The listing builds one solid part. Answer for the finished solid, in the listing's coordinates (mm). A direction names the side the tool comes from. Give positions to 0.01 mm unless a question says otherwise; leave off trailing zeros. Order: outer loops, then holes, each group sorted by start corner. A loop starts at its lowest first (then second) coordinate and runs counter-clockwise, first axis right, second up. Notation, with made-up numbers: (29.25, -29) - (73.25, -29) arc R20 cw to (73.25, -19) - close; hole circle Ø4 at (30, 65). An arc over 180 degrees is marked (long way). Use CSV: the item, a comma, the result in double quotes.
```python
from build123d import *

# Parameters (mm, degrees)
SKETCH1_W               = 140
SKETCH1_H               = 60
BOSS_EXTRUDE1_DEPTH     = 5
SKETCH2_W               = 140
SKETCH2_H               = 5
BOSS_EXTRUDE3_DEPTH     = 50
SKETCH4_R               = 7
CUT_EXTRUDE1_DEPTH      = 108.354552768
SKETCH5_W               = 50
SKETCH5_H               = 50
SKETCH5_W_2             = 40
SKETCH5_H_2             = 40
BOSS_EXTRUDE4_DEPTH     = 1015
CUT_EXTRUDE3_DEPTH      = 2088.648198332
CUT_EXTRUDE3_DEPTH_BACK = 2088.648198332


with BuildPart() as part:
    # Sketch1 → Boss-Extrude1 (new body)
    with BuildSketch(Plane(origin=(0, 0, 0), x_dir=(1, 0, 0), z_dir=(0, 1, 0))):
        with Locations((0, 15)):
            Rectangle(SKETCH1_W, SKETCH1_H)
    extrude(amount=-BOSS_EXTRUDE1_DEPTH)

    # Sketch2 → Boss-Extrude3 (add)
    with BuildSketch(Plane.XZ.offset(5)):
        with Locations((0, 12.5)):
            Rectangle(SKETCH2_W, SKETCH2_H)
        with Locations((0, -42.5)):
            Rectangle(SKETCH2_W, SKETCH2_H)
    extrude(amount=BOSS_EXTRUDE3_DEPTH)

    # Sketch4 → Cut-Extrude1 (cut, through all)
    with BuildSketch(Plane.XY.offset(15)):
        with Locations((-45, -27.5)):
            Circle(SKETCH4_R)
        with Locations((45, -27.5)):
            Circle(SKETCH4_R)
    extrude(amount=-CUT_EXTRUDE1_DEPTH, mode=Mode.SUBTRACT)

    # Sketch5 → Boss-Extrude4 (add)
    with BuildSketch(Plane(origin=(0, 0, 0), x_dir=(1, 0, 0), z_dir=(0, 1, 0))):
        with Locations((0, 15)):
            Rectangle(SKETCH5_W, SKETCH5_H)
        with Locations((0, 15)):
            Rectangle(SKETCH5_W_2, SKETCH5_H_2, mode=Mode.SUBTRACT)
    extrude(amount=BOSS_EXTRUDE4_DEPTH)

    # Mirror1: part across plane


with BuildPart() as part_1:
    add(part.part)
    add(part.part.mirror(Plane.ZX.offset(1015)))

    # Sketch8 → Cut-Extrude3 (cut, two sides: drawn at the far end of the back side and taken through both)
    with BuildSketch(Plane.ZY.offset(25).offset(-CUT_EXTRUDE3_DEPTH_BACK)):
        with BuildLine():
            Line((-32.587539874, 2030), (-32.587539874, 1955.085156016))
            ThreePointArc((-32.587539874, 1955.085156016), (-16.293769937, 1938.791386079), (0, 1955.085156016))
            Line((0, 1955.085156016), (0, 2030))
            Line((0, 2030), (-32.587539874, 2030))
        make_face()
    extrude(amount=CUT_EXTRUDE3_DEPTH + CUT_EXTRUDE3_DEPTH_BACK, mode=Mode.SUBTRACT)


solid = part_1.part
```
Item 1: The part is cut by section B-B (z = -17). Give the vertices of the cut face in (x, y), and give its area (3 significant figures).
Taken from the geometry:
outline,"(-70, -5) - (70, -5) - (70, 0) - (25, 0) - (25, 1938.81) - (20, 1938.81) - (20, 0) - (-20, 0) - (-20, 1938.81) - (-25, 1938.81) - (-25, 0) - (-70, 0) - close; (-70, 2030) - (70, 2030) - (70, 2035) - (-70, 2035) - close"
area,"20,800 mm^2"
Item 2: Find the intervals of material crossed by line 1 along Y through (x, z) = (-45, 12.45); line 2 along Z through (x, y) = (-8.5, 1957); line 3 along X through (y, z) = (736, -33), in increasing order.
Taken from the geometry:
line 1,"-55 to -34.5, -20.5 to 0, 2030 to 2050.5, 2064.5 to 2085"
line 2,"-40 to -35, 5 to 10"
line 3,"-25 to -20, 20 to 25"
Item 3: Each of these flat-tipped pins is pushed along its axis until it touches: pin 1 (8.5 mm diameter, centred on x = 45, y = -27.5, fed in from -Z); pin 2 (1.5 mm diameter, centred on x = -23.5, y = 1982, fed in from -Z); pin 3 (1.5 mm diameter, centred on x = -7.5, z = 1.5, fed in from +Y); pin 4 (2 mm diameter, centred on y = 528, z = -13.5, fed in from +X). Where does it stop, or does it pass through?
Taken from the geometry:
pin 1,"through"
pin 2,"z = -40"
pin 3,"y = 2035"
pin 4,"x = 25"
Item 4: The part is cut by section A-A (y = 1279.5). Give the vertices of the cut face in (x, z).
Taken from the geometry:
outline,"(-25, -40) - (25, -40) - (25, 10) - (-25, 10) - close; hole (-20, -35) - (20, -35) - (20, 5) - (-20, 5) - close"
Item 5: The mould has two halves that part along Z. Classify faces 4 (the face through (-1, 0, 11)), 5 (the face through (-1, -30, 10)), 6 (the face through (0, 1029, -40)), 7 (the face through (-1, -27, 15)): +Z half, -Z half, draft (parallel to the pull), parting line (faces both ways), or undercut.
Taken from the geometry:
face 4,"draft"
face 5,"undercut"
face 6,"-Z half"
face 7,"+Z half"
Item 6: Which of the six approach directions +Z, -Z, +X, -X, +Y, -Y give full straight-line access (tool end or side, diameter ignored) to faces 1 (the face through (-1, -30, -40)), 2 (the face through (-1, 2060, 10)), 3 (the face through (-25, 1029, -15))?
Taken from the geometry:
face 1,"+X, -X, -Y"
face 2,"+X, -X, +Y"
face 3,"+Z, -Z, -X"
